Geometry check sheet. Reference: the model listing, model coordinates, mm. Round coordinates to 2 decimals unless told otherwise and drop trailing zeros.
(1) Gauge pin test, flat ends, axial feed: P1, Ø3, axis at x = 134, z = 12.5, coming from the +Y side; P2, Ø10, axis at y = 149, z = 12, coming from the -X side; P3, Ø3, axis at y = 164, z = 15.5, coming from the +X side. Record the tip position at first contact, or that the pin passes through.
(2) Cross-section at A-A on x = 110.5. Count the separate pieces of the cut face and the enclosed holes in it, and give its area (3 significant figures).
(3) Thickness scan on L1, parallel to Y at x = 88, z = 5.25; L2, parallel to Y at x = 193, z = 5.75; L3, parallel to X at y = 78, z = 22.25. Record the ranges inside material, lowest first.
(4) Draft check along Y on faces 1 (the face through (100.566, 153.337, 13.868)), 2 (the face through (99, 127, 25.4)). Enter one of: pulls with the +Y half, pulls with the -Y half, needs draft (parallel to the pull), parting line crosses it, or undercut.
from build123d import *

# Parameters (mm, degrees)
F0_W     = 203.2
F0_H     = 254
F0_R     = 25.4
F1_DEPTH = 25.4
F1_TAPER = -3
F2_R     = 6.35


with BuildPart() as f1:
    # F0 (on Top) → F1 (new body)
    with BuildSketch(Plane.XY):
        with Locations((101.6, 127)):
            Rectangle(F0_W, F0_H)
        with Locations((103.7775874138, 76.2)):
            Circle(F0_R, mode=Mode.SUBTRACT)
        with Locations((103.7775874138, 177.8)):
            Circle(F0_R, mode=Mode.SUBTRACT)
    extrude(amount=F1_DEPTH, taper=F1_TAPER)

    # F2
    f2_edges = [f1.edges().sort_by_distance(p)[0] for p in [
        (0, 127, 0),
        (-1.331158, 127, 25.4),
        (-0.665579, 254.665579, 12.7),
        (101.6, 255.331158, 25.4),
        (79.708745, 177.8, 25.4),
        (78.377587, 177.8, 0),
        (128.512009, 177.8, 12.7),
        (-0.665579, -0.665579, 12.7),
        (101.6, -1.331158, 25.4),
        (204.531158, 127, 25.4),
        (79.708745, 76.2, 25.4),
        (78.377587, 76.2, 0),
        (128.512009, 76.2, 12.7),
        (101.6, 0, 0),
        (203.865579, -0.665579, 12.7),
        (101.6, 254, 0),
        (203.2, 127, 0),
        (203.865579, 254.665579, 12.7),
    ]]
    fillet(f2_edges, radius=F2_R)


solid = f1.part
Found:
1. P1: stops at y = 254.73
1. P2: stops at x = -0.89
1. P3: stops at x = 204.09
2. separate pieces: 3
2. enclosed holes: 0
2. area: 3,960 mm2
3. L1: y = -0.23 to 56.59, 95.81 to 158.19, 197.41 to 254.23
3. L2: y = -0.3 to 254.3
3. L3: x = -0.12 to 78.57, 128.99 to 203.32
4. face 1: undercut
4. face 2: needs draft
